Here's how the part is built. I have some questions about the finished solid (model axes, mm). A direction names the side the tool comes from. Round coordinates to 2 decimals unless told otherwise and drop trailing zeros. Loops run counter-clockwise (first coordinate to the right, second up) from the corner with the lowest first, then second, coordinate; pieces in that order, holes last. Notation, with made-up numbers: M 44,59.25 L 83,59.25 A31 cw 83,88.25 Z; hole C -29,48.25 d8. An arc over 180 degrees is marked long. Use a Markdown table: item, result.
from build123d import *

# Parameters (mm, degrees)
BOSS_EXTRUDE1_DEPTH = 1.524


with BuildPart() as part:
    # Sketch1 → Boss-Extrude1 (new body)
    with BuildSketch(Plane.XY):
        with BuildLine():
            Line((0.285426682, 0), (0.285426682, -1.524))
            Line((0.285426682, -1.524), (10.508401923, -1.524))
            ThreePointArc((10.508401923, -1.524), (9.401321759, -4.352342754), (9.024565628, -7.366178191))
            ThreePointArc((9.024565628, -7.366178191), (5.632541896, -10.599139275), (1.353650751, -12.509362545))
            ThreePointArc((1.353650751, -12.509362545), (-2.688908753, -13.751919893), (-6.559224402, -15.456881148))
            ThreePointArc((-6.559224402, -15.456881148), (-6.892797133, -14.362674131), (-7.1651622, -13.251648913))
            Line((-7.1651622, -13.251648913), (-0.813548275, -11.074651995))
            Line((-0.813548275, -11.074651995), (-1.307676516, -9.632981686))
            Line((-1.307676516, -9.632981686), (-7.434081645, -11.732788954))
            ThreePointArc((-7.434081645, -11.732788954), (-7.444704809, -6.146254485), (-5.954978709, -0.762))
            ThreePointArc((-5.954978709, -0.762), (-7.444704809, 4.622254485), (-7.434081645, 10.208788954))
            Line((-7.434081645, 10.208788954), (-1.307676516, 8.108981686))
            Line((-1.307676516, 8.108981686), (-0.813548275, 9.550651995))
            Line((-0.813548275, 9.550651995), (-7.1651622, 11.727648913))
            ThreePointArc((-7.1651622, 11.727648913), (-6.892797133, 12.838674131), (-6.559224402, 13.932881148))
            ThreePointArc((-6.559224402, 13.932881148), (-2.688908753, 12.227919893), (1.353650751, 10.985362545))
            ThreePointArc((1.353650751, 10.985362545), (5.632541896, 9.075139275), (9.024565628, 5.842178191))
            ThreePointArc((9.024565628, 5.842178191), (9.401321759, 2.828342754), (10.508401923, 0))
            Line((10.508401923, 0), (0.285426682, 0))
        make_face()
    extrude(amount=BOSS_EXTRUDE1_DEPTH)


solid = part.part
1. For pin 1 Ø1 at (x, y) = (-4, 5.5) entering from -Z; pin 2 Ø0.5 at (x, z) = (3, 1) entering from +Y, each with a flat end and sliding along its axis, tell me the tip position at first contact or that it passes through.
Answer sheet:
| item | result |
|---|---|
| pin 1 | z = 0 |
| pin 2 | y = 10.55 |
2. We'd pull the mould along X, two halves only. Please class faces 4 (the face through (-2.63, -13.73, 0.75)), 5 (the face through (-7.455, -6.224, 0.751)), 6 (the face through (-4.33, -10.67, 0.75)), 7 (the face through (5, -1.524, 1)): +X half, -X half, draft (parallel to the pull), parting line (faces both ways), or undercut.
Answer sheet:
| item | result |
|---|---|
| face 4 | +X half |
| face 5 | -X half |
| face 6 | undercut |
| face 7 | draft |
3. Imagine slicing it at B-B, the plane z = 0.35. Write out the boundary of the cut face in (x, y).
Answer sheet:
| item | result |
|---|---|
| outline | M -7.43,-11.73 L -1.31,-9.63 L -0.81,-11.07 L -7.17,-13.25 A20.61 ccw -6.56,-15.46 A36.25 cw 1.35,-12.51 A13.79 ccw 9.02,-7.37 A12.24 cw 10.51,-1.52 L 0.29,-1.52 L 0.29,0 L 10.51,0 A12.24 cw 9.02,5.84 A13.79 ccw 1.35,10.99 A36.25 cw -6.56,13.93 A20.61 ccw -7.17,11.73 L -0.81,9.55 L -1.31,8.11 L -7.43,10.21 A20.61 ccw -5.95,-0.76 A20.61 ccw Z |
4. Which directions (+Z, -Z, +X, -X, +Y, -Y) give clear straight access to the entire face, cutting with the end or side of a thin tool? Please do faces 1 (the face through (-4.034, -12.178, 0.751)), 2 (the face through (0.285, -1, 1)), 3 (the face through (5.58, 9.11, 0.75)).
Answer sheet:
| item | result |
|---|---|
| face 1 | +Z, -Z |
| face 2 | +Z, -Z, +X |
| face 3 | +Z, -Z, +X, +Y |
5. Imagine slicing it at A-A, the plane x = 5.25. Write out the boundary of the cut face in (y, z), then the cut area to 3 significant figures.
Answer sheet:
| item | result |
|---|---|
| outline | M -10.85,0 L -1.52,0 L -1.52,1.52 L -10.85,1.52 Z; M 0,0 L 9.32,0 L 9.32,1.52 L 0,1.52 Z |
| area | 28.4 mm2 |
6. I need wall thicknesses on probe 1 along Y at (x, z) = (-1.5, 0.3); probe 2 along Y at (x, z) = (-5.5, 1); probe 3 along Y at (x, z) = (3.75, 0.7). Which ranges of each line are inside material? Lowest first, please. Write a range as from..to.
Answer sheet:
| item | result |
|---|---|
| probe 1 | -13.33..-11.31, -9.7..8.17, 9.79..11.81 |
| probe 2 | -14.94..-12.68, -11.07..9.55, 11.16..13.41 |
| probe 3 | -11.66..-1.52, 0..10.13 |
7. Imagine slicing it at C-C, the plane x = -3.25. Write out the boundary of the cut face in (y, z).
Answer sheet:
| item | result |
|---|---|
| outline | M -13.97,0 L -11.91,0 L -11.91,1.52 L -13.97,1.52 Z; M -10.3,0 L 8.77,0 L 8.77,1.52 L -10.3,1.52 Z; M 10.39,0 L 12.44,0 L 12.44,1.52 L 10.39,1.52 Z |
8. Imagine slicing it at D-D, the plane x = 1. Write out the boundary of the cut face in (y, z), then the cut area to 3 significant figures.
Answer sheet:
| item | result |
|---|---|
| outline | M -12.6,0 L -1.52,0 L -1.52,1.52 L -12.6,1.52 Z; M 0,0 L 11.07,0 L 11.07,1.52 L 0,1.52 Z |
| area | 33.8 mm2 |
